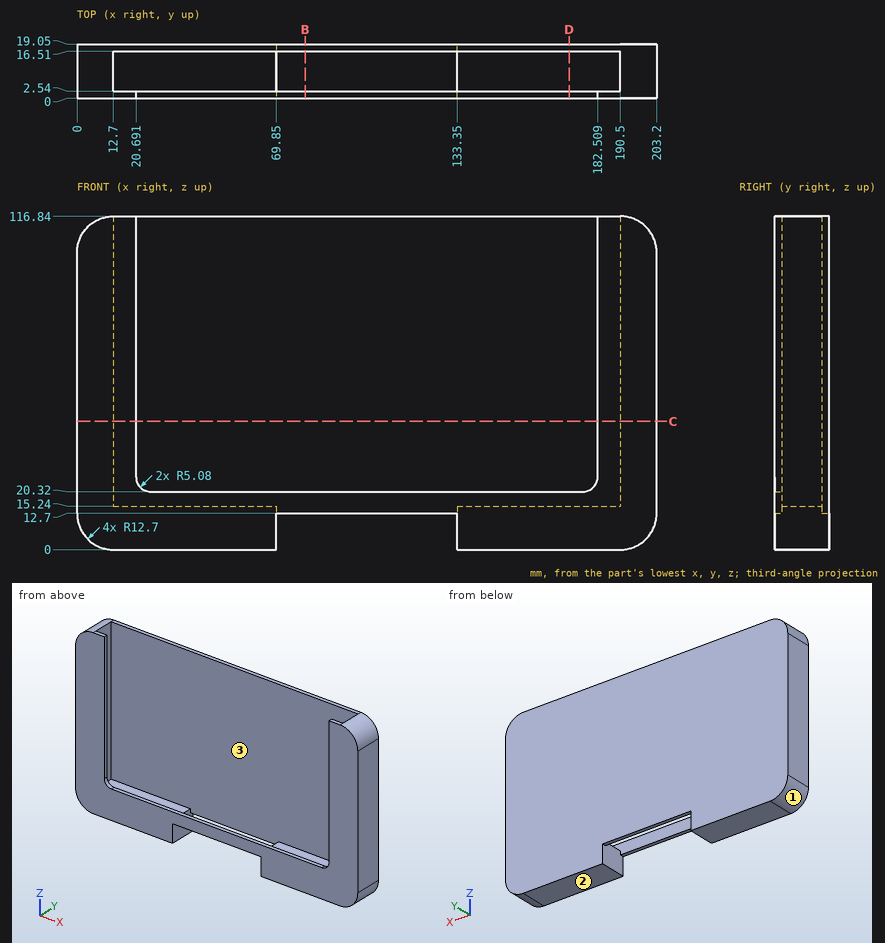
Geometry: see drawing. Coordinates: mm, zero at the bounding-box minimum. Coordinates: 2 decimals unless noted, no trailing zeros. Loops run counter-clockwise (first coordinate to the right, second up) from the corner with the lowest first, then second, coordinate; pieces in that order, holes last. Notation, with made-up numbers: (68, 2.25) -> (94, 2.25) arc R3 ccw to (94, 7.25) -> close; hole circle Ø4 at (60, -24). An arc over 180 degrees is marked (long way). Write item = value, one per line. Start each with the question number.
Item 1: Cut plane D-D, the plane x = 172.5. Return loops of the section in (y, z), plus the area to 3 significant figures.
Item 2: Cut plane B-B, the plane x = 80. Return loops of the section in (y, z), plus the area to 3 significant figures.
Item 3: First-contact query: P1, Ø1.5, axis at x = 159.5, y = 15.5, coming from the +Z side; P2, Ø0.8, axis at x = 88.5, y = 1, coming from the +Z side; P3, Ø3, axis at x = 105, y = 17.5, coming from the -Z side. Flat tips, straight axial feed; report the tip coordinate or a pass-through.
Item 4: Mould query, pull axis X, two halves, no side actions, for the marked faces 1, 2 and 3. Classes: pulls with the +X half, pulls with the -X half, needs draft (parallel to the pull), parting line crosses it, or undercut.
Item 5: Material intervals for line 1 (X direction, y = 9, z = 32); line 2 (Y direction, x = 27, z = 17); line 3 (X direction, y = 1.5, z = 44), sorted ascending.
Item 6: Cut plane C-C, the plane z = 45. Return loops of the section in (x, y).
Ans:
q1.outline = (0, 0) -> (19.05, 0) -> (19.05, 116.84) -> (16.51, 116.84) -> (16.51, 15.24) -> (2.54, 15.24) -> (2.54, 20.32) -> (0, 20.32) -> close
q1.area = 561 mm²
q2.outline = (0, 12.7) -> (2.54, 12.7) -> (2.54, 20.32) -> (0, 20.32) -> close; (16.51, 12.7) -> (19.05, 12.7) -> (19.05, 116.84) -> (16.51, 116.84) -> close
q2.area = 284 mm²
q3.P1 = 15.24
q3.P2 = 20.32
q3.P3 = 12.7
q4.face_1 = pulls with the -X half
q4.face_2 = needs draft
q4.face_3 = undercut
q5.line_1 = 0 to 12.7, 190.5 to 203.2
q5.line_2 = 0 to 2.54, 16.51 to 19.05
q5.line_3 = 0 to 20.69, 182.51 to 203.2
q6.outline = (0, 0) -> (20.69, 0) -> (20.69, 2.54) -> (12.7, 2.54) -> (12.7, 16.51) -> (190.5, 16.51) -> (190.5, 2.54) -> (182.51, 2.54) -> (182.51, 0) -> (203.2, 0) -> (203.2, 19.05) -> (0, 19.05) -> close
